Here's how the part is built. I have some questions about the finished solid (model axes, mm). Round coordinates to 2 decimals unless told otherwise and drop trailing zeros. Order: outer loops, then holes, each group sorted by start corner. A loop starts at its lowest first (then second) coordinate and runs counter-clockwise, first axis right, second up. Notation, with made-up numbers: (3.5, -33) - (27.5, -33) arc R29 cw to (27.5, -13) - close; hole circle Ø11 at (24, -26). An arc over 180 degrees is marked (long way). One line per item, written item: value.
from build123d import *

# Parameters (mm, degrees)
SKETCH1_R             = 87.5
BOSS_EXTRUDE1_DEPTH   = 24
SKETCH2_R             = 7.5
CUT_EXTRUDE1_DEPTH    = 127.049593415
SKETCH3_R             = 7.120707896
CUT_EXTRUDE2_DEPTH    = 22.318548
CIRPATTERN1_START     = 1.681451558
CIRPATTERN1_OUTLINE_R = 7.120707896
CIRPATTERN1_DEPTH     = 22.318548442


# Read off the part's stored shape, not the designer's step: CirPattern1
with BuildPart() as part:
    # Sketch1 → Boss-Extrude1 (new body)
    with BuildSketch(Plane(origin=(0, 0, 0), x_dir=(1, 0, 0), z_dir=(0, 1, 0))):
        with Locations(Location((0, 0, 0), (0, 0, 270))):
            Circle(SKETCH1_R)
    extrude(amount=BOSS_EXTRUDE1_DEPTH)

    # Sketch2 → Cut-Extrude1 (cut, through all)
    with BuildSketch(Plane(origin=(0, 0, 0), x_dir=(1, 0, 0), z_dir=(0, 1, 0))):
        with Locations(Location((0, 0, 0), (0, 0, 270))):
            Circle(SKETCH2_R)
    extrude(amount=CUT_EXTRUDE1_DEPTH, mode=Mode.SUBTRACT)

    # Sketch3 → Cut-Extrude2 (cut)
    with BuildSketch(Plane(origin=(0, 24, 0), x_dir=(1, 0, 0), z_dir=(0, 1, 0))):
        with Locations(Location((-34.52893475, 0, 0), (0, 0, 270))):
            Circle(SKETCH3_R)
    extrude(amount=-CUT_EXTRUDE2_DEPTH, mode=Mode.SUBTRACT)

    # CirPattern1 outline → CirPattern1 (cut)
    with BuildSketch(Plane(origin=(0, 0, 0), x_dir=(1, 0, 0), z_dir=(0, 1, 0)).offset(CIRPATTERN1_START)):
        with Locations((-10.670027635, -32.838968394)):
            Circle(CIRPATTERN1_OUTLINE_R)
        with Locations((27.93449501, -20.295598623)):
            Circle(CIRPATTERN1_OUTLINE_R)
        with Locations((27.93449501, 20.295598623)):
            Circle(CIRPATTERN1_OUTLINE_R)
        with Locations((-10.670027635, 32.838968394)):
            Circle(CIRPATTERN1_OUTLINE_R)
    extrude(amount=CIRPATTERN1_DEPTH, mode=Mode.SUBTRACT)


solid = part.part
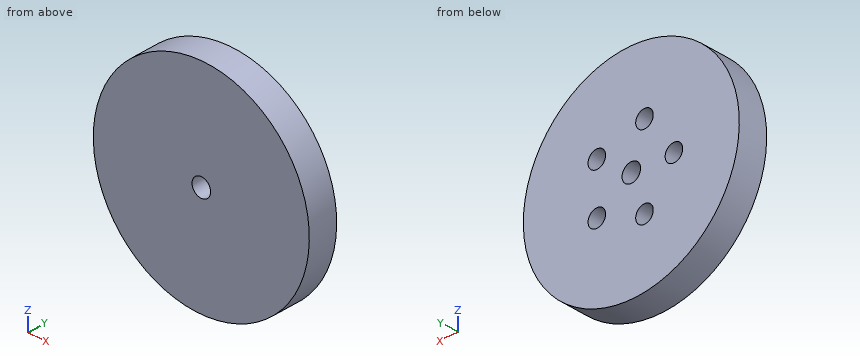
Q1. If we section it at D-D, the plane z = 29.5: Please give me the cut outline in (x, y).
Results list:
outline: (-82.38, 0) - (82.38, 0) - (82.38, 24) - (-4.38, 24) - (-4.38, 1.68) - (-16.96, 1.68) - (-16.96, 24) - (-82.38, 24) - close
Q2. If we section it at C-C, the plane y = 9.5: Please give me the cut outline in (x, z).
Results list:
outline: circle Ø175 at (0, 0); hole circle Ø14.24 at (-34.53, 0); hole circle Ø14.24 at (-10.67, -32.84); hole circle Ø14.24 at (-10.67, 32.84); hole circle Ø15 at (0, 0); hole circle Ø14.24 at (27.93, -20.3); hole circle Ø14.24 at (27.93, 20.3)
Q3. If we section it at B-B, the plane x = 0: Please give me the cut outline in (y, z).
Results list:
outline: (0, -87.5) - (24, -87.5) - (24, -7.5) - (0, -7.5) - close; (0, 7.5) - (24, 7.5) - (24, 87.5) - (0, 87.5) - close
Q4. Will these pins go through, and if not, where does the flat tip stop? pin 1 (10 mm diameter, centred on x = -29, y = 15.5, fed in from +Z); pin 2 (6 mm diameter, centred on y = 3.5, z = -51.5, fed in from -X); pin 3 (10 mm diameter, centred on x = 8.5, y = 17, fed in from -Z).
Results list:
pin 1: z = 84.14
pin 2: x = -72.83
pin 3: z = -87.43
Q5. If I drill on line 1 along X through (y, z) = (11.25, 0); line 2 along Z through (x, y) = (-9, 4.5); line 3 along Y through (x, z) = (-11.5, 27), over which ranges is the centre line in solid material (lowest first)?
Results list:
line 1: -87.5 to -41.65, -27.41 to -7.5, 7.5 to 87.5
line 2: -87.04 to -39.76, -25.92 to 25.92, 39.76 to 87.04
line 3: 0 to 1.68
Q6. If we section it at A-A, the plane z = 0: Please give me the cut outline in (x, y).
Results list:
outline: (-87.5, 0) - (-7.5, 0) - (-7.5, 24) - (-27.41, 24) - (-27.41, 1.68) - (-41.65, 1.68) - (-41.65, 24) - (-87.5, 24) - close; (7.5, 0) - (87.5, 0) - (87.5, 24) - (7.5, 24) - close
